from build123d import *

# Parameters (mm, degrees)
CROQUIS2_W              = 290
CROQUIS2_H              = 130
SALIENTE_EXTRUIR1_DEPTH = 5
CROQUIS3_W              = 90
CROQUIS3_H              = 5
CORTAR_EXTRUIR1_DEPTH   = 159.981130956
CROQUIS4_W              = 20.5
CROQUIS4_H              = 25.7
CORTAR_EXTRUIR2_DEPTH   = 4
CROQUIS5_R              = 1.25
CORTAR_EXTRUIR3_DEPTH   = 4
CROQUIS6_W              = 92
CROQUIS6_H              = 104.5
CORTAR_EXTRUIR4_DEPTH   = 3
CROQUIS7_W              = 100
CROQUIS7_H              = 8.5
CORTAR_EXTRUIR5_DEPTH   = 159.981130956
CROQUIS8_R              = 2
CORTAR_EXTRUIR6_DEPTH   = 159.981130956
CROQUIS9_R              = 3.75
CORTAR_EXTRUIR7_DEPTH   = 2
CROQUIS10_W             = 122
CROQUIS10_H             = 82
CORTAR_EXTRUIR8_DEPTH   = 4
CROQUIS13_R             = 1.4
CORTAR_EXTRUIR9_DEPTH   = 3
CROQUIS14_R             = 1.4
CORTAR_EXTRUIR10_DEPTH  = 3
SALIENTE_EXTRUIR2_DEPTH = 1
CROQUIS16_R             = 1.375
CORTAR_EXTRUIR11_DEPTH  = 159.95282319


with BuildPart() as part:
    # Croquis2 → Saliente-Extruir1 (new body)
    with BuildSketch(Plane(origin=(0, 0, 0), x_dir=(1, 0, 0), z_dir=(0, 1, 0))):
        Rectangle(CROQUIS2_W, CROQUIS2_H)
    extrude(amount=SALIENTE_EXTRUIR1_DEPTH)

    # Croquis3 → Cortar-Extruir1 (cut, through all)
    with BuildSketch(Plane(origin=(0, 5, 0), x_dir=(1, 0, 0), z_dir=(0, 1, 0))):
        with Locations((92.5, -57.5)):
            Rectangle(CROQUIS3_W, CROQUIS3_H)
        with Locations((-92.5, -57.5)):
            Rectangle(CROQUIS3_W, CROQUIS3_H)
        with Locations((92.5, 57.5)):
            Rectangle(CROQUIS3_W, CROQUIS3_H)
        with Locations((-92.5, 57.5)):
            Rectangle(CROQUIS3_W, CROQUIS3_H)
    extrude(amount=-CORTAR_EXTRUIR1_DEPTH, mode=Mode.SUBTRACT)

    # Croquis4 → Cortar-Extruir2 (cut)
    with BuildSketch(Plane(origin=(0, 5, 0), x_dir=(1, 0, 0), z_dir=(0, 1, 0))):
        with Locations((-120.05, -1.95)):
            Rectangle(CROQUIS4_W, CROQUIS4_H)
    extrude(amount=-CORTAR_EXTRUIR2_DEPTH, mode=Mode.SUBTRACT)

    # Croquis5 → Cortar-Extruir3 (cut)
    with BuildSketch(Plane(origin=(0, 1, 0), x_dir=(1, 0, 0), z_dir=(0, 1, 0))):
        with Locations(Location((-127.8, 8.4, 0), (0, 0, 270))):
            Circle(CROQUIS5_R)
        with Locations(Location((-112.3, 8.4, 0), (0, 0, 90))):
            Circle(CROQUIS5_R)
        with Locations(Location((-112.3, -12.3, 0), (0, 0, 270))):
            Circle(CROQUIS5_R)
        with Locations(Location((-127.8, -12.3, 0), (0, 0, 90))):
            Circle(CROQUIS5_R)
    extrude(amount=-CORTAR_EXTRUIR3_DEPTH, mode=Mode.SUBTRACT)

    # Croquis6 → Cortar-Extruir4 (cut)
    with BuildSketch(Plane(origin=(0, 5, 0), x_dir=(1, 0, 0), z_dir=(0, 1, 0))):
        with Locations((85.8, 0)):
            Rectangle(CROQUIS6_W, CROQUIS6_H)
    extrude(amount=-CORTAR_EXTRUIR4_DEPTH, mode=Mode.SUBTRACT)

    # Croquis7 → Cortar-Extruir5 (cut, through all)
    with BuildSketch(Plane(origin=(0, 5, 0), x_dir=(1, 0, 0), z_dir=(0, 1, 0))):
        with Locations((-50, -46.25)):
            Rectangle(CROQUIS7_W, CROQUIS7_H)
        with Locations((-50, 46.25)):
            Rectangle(CROQUIS7_W, CROQUIS7_H)
    extrude(amount=-CORTAR_EXTRUIR5_DEPTH, mode=Mode.SUBTRACT)

    # Croquis8 → Cortar-Extruir6 (cut, through all)
    with BuildSketch(Plane(origin=(0, 5, 0), x_dir=(1, 0, 0), z_dir=(0, 1, 0))):
        with Locations(Location((-140, 50, 0), (0, 0, 270))):
            Circle(CROQUIS8_R)
        with Locations(Location((140, 50, 0), (0, 0, 90))):
            Circle(CROQUIS8_R)
        with Locations(Location((140, -50, 0), (0, 0, 270))):
            Circle(CROQUIS8_R)
        with Locations(Location((-140, -50, 0), (0, 0, 90))):
            Circle(CROQUIS8_R)
    extrude(amount=-CORTAR_EXTRUIR6_DEPTH, mode=Mode.SUBTRACT)

    # Croquis9 → Cortar-Extruir7 (cut)
    with BuildSketch(Plane(origin=(0, 5, 0), x_dir=(1, 0, 0), z_dir=(0, 1, 0))):
        with Locations(Location((-140, 50, 0), (0, 0, 270))):
            Circle(CROQUIS9_R)
        with Locations(Location((-140, -50, 0), (0, 0, 90))):
            Circle(CROQUIS9_R)
        with Locations(Location((140, -50, 0), (0, 0, 270))):
            Circle(CROQUIS9_R)
        with Locations(Location((140, 50, 0), (0, 0, 90))):
            Circle(CROQUIS9_R)
    extrude(amount=-CORTAR_EXTRUIR7_DEPTH, mode=Mode.SUBTRACT)

    # Croquis10 → Cortar-Extruir8 (cut)
    with BuildSketch(Plane(origin=(0, 5, 0), x_dir=(1, 0, 0), z_dir=(0, 1, 0))):
        with Locations((-46.8, 0)):
            Rectangle(CROQUIS10_W, CROQUIS10_H)
    extrude(amount=-CORTAR_EXTRUIR8_DEPTH, mode=Mode.SUBTRACT)

    # Croquis13 → Cortar-Extruir9 (cut)
    with BuildSketch(Plane(origin=(0, 1, 0), x_dir=(1, 0, 0), z_dir=(0, 1, 0))):
        with Locations(Location((-104.3, 37.5, 0), (0, 0, 270))):
            Circle(CROQUIS13_R)
        with Locations(Location((10.7, 37.5, 0), (0, 0, 90))):
            Circle(CROQUIS13_R)
        with Locations(Location((10.7, -37.5, 0), (0, 0, 270))):
            Circle(CROQUIS13_R)
        with Locations(Location((-104.3, -37.5, 0), (0, 0, 90))):
            Circle(CROQUIS13_R)
    extrude(amount=-CORTAR_EXTRUIR9_DEPTH, mode=Mode.SUBTRACT)

    # Croquis14 → Cortar-Extruir10 (cut)
    with BuildSketch(Plane(origin=(0, 1, 0), x_dir=(1, 0, 0), z_dir=(0, 1, 0))):
        with Locations(Location((-104.3, -37.5, 0), (0, 0, 90))):
            Circle(CROQUIS14_R)
        with Locations(Location((-104.3, 37.5, 0), (0, 0, 270))):
            Circle(CROQUIS14_R)
        with Locations(Location((-11.3, 37.5, 0), (0, 0, 90))):
            Circle(CROQUIS14_R)
        with Locations(Location((-11.3, -37.5, 0), (0, 0, 90))):
            Circle(CROQUIS14_R)
    extrude(amount=-CORTAR_EXTRUIR10_DEPTH, mode=Mode.SUBTRACT)

    # Croquis15 → Saliente-Extruir2 (add)
    with BuildSketch(Plane(origin=(0, 5, 0), x_dir=(1, 0, 0), z_dir=(0, 1, 0))):
        with BuildLine():
            Line((-107.8, 42), (-100.783894533, 42))
            Line((-100.783894533, 42), (-100.783894533, 41))
            Line((-100.783894533, 41), (-107.8, 41))
            Line((-107.8, 41), (-107.8, 34.318360621))
            Line((-107.8, 34.318360621), (-108.8, 34.318360621))
            Line((-108.8, 34.318360621), (-108.8, 41))
            ThreePointArc((-108.8, 41), (-108.507106781, 41.707106781), (-107.8, 42))
        make_face()
        with BuildLine():
            Line((15.2, 41), (15.2, 34.318360621))
            Line((15.2, 34.318360621), (14.2, 34.318360621))
            Line((14.2, 34.318360621), (14.2, 41))
            Line((14.2, 41), (7.183894533, 41))
            Line((7.183894533, 41), (7.183894533, 42))
            Line((7.183894533, 42), (14.2, 42))
            ThreePointArc((14.2, 42), (14.907106781, 41.707106781), (15.2, 41))
        make_face()
        with BuildLine():
            Line((14.2, -42), (7.183894533, -42))
            Line((7.183894533, -42), (7.183894533, -41))
            Line((7.183894533, -41), (14.2, -41))
            Line((14.2, -41), (14.2, -34.318360621))
            Line((14.2, -34.318360621), (15.2, -34.318360621))
            Line((15.2, -34.318360621), (15.2, -41))
            ThreePointArc((15.2, -41), (14.907106781, -41.707106781), (14.2, -42))
        make_face()
        with BuildLine():
            Line((-108.8, -41), (-108.8, -34.318360621))
            Line((-108.8, -34.318360621), (-107.8, -34.318360621))
            Line((-107.8, -34.318360621), (-107.8, -41))
            Line((-107.8, -41), (-100.783894533, -41))
            Line((-100.783894533, -41), (-100.783894533, -42))
            Line((-100.783894533, -42), (-107.8, -42))
            ThreePointArc((-107.8, -42), (-108.507106781, -41.707106781), (-108.8, -41))
        make_face()
    extrude(amount=SALIENTE_EXTRUIR2_DEPTH)

    # Croquis16 → Cortar-Extruir11 (cut, through all)
    with BuildSketch(Plane(origin=(0, 2, 0), x_dir=(1, 0, 0), z_dir=(0, 1, 0))):
        with Locations(Location((50.3, 40, 0), (0, 0, 270))):
            Circle(CROQUIS16_R)
        with Locations(Location((50.3, -46, 0), (0, 0, 270))):
            Circle(CROQUIS16_R)
        with Locations(Location((108.3, 40, 0), (0, 0, 270))):
            Circle(CROQUIS16_R)
        with Locations(Location((108.3, -46, 0), (0, 0, 270))):
            Circle(CROQUIS16_R)
    extrude(amount=-CORTAR_EXTRUIR11_DEPTH, mode=Mode.SUBTRACT)


solid = part.part
Can you work these out from the model? Positions are in its coordinate system, mm. A direction names the side the tool comes from. Coordinates: 2 decimals unless noted, no trailing zeros. Loops run counter-clockwise (first coordinate to the right, second up) from the corner with the lowest first, then second, coordinate; pieces in that order, holes last. Notation, with made-up numbers: M 83.25,-24 L 117.25,-24 A33 cw 117.25,10 Z; hole C 17,60.5 d2. An arc over 180 degrees is marked long. Return JSON: item names as keys, results as strings. Group by question number.
Item 1: On a 3-axis mill with a long thin cutter (end or side, diameter ignored), from which of +Z, -Z, +X, -X, +Y, -Y can I reach the whole of each face in a straight line? I mean faces 1 (the flat face through (-107.8, 3, 1)), 2 (the flat face through (-2, 2, -65)), 3 (the flat face through (-100, 3, 46)). Say none if no direction works.
Item 2: Imagine slicing it at C-C (z = -24.5). Please give me the cut outline in (x, y).
Item 3: Imagine slicing it at A-A (x = -16). Please give me the cut outline in (y, z), and give its area (3 significant figures).
Item 4: Imagine slicing it at B-B (z = 3.5). Please give me the cut outline in (x, y), and give its area (3 significant figures).
Item 5: I'm going to push flat-ended pins straight in: pin 1 Ø4.5 at (x, z) = (-104.3, 37.5) entering from -Y; pin 2 Ø0.8 at (y, z) = (5.5, 41.5) entering from -X (3 decimals); pin 3 Ø3.5 at (x, z) = (-104.3, -37.5) entering from +Y; pin 4 Ø7 at (x, z) = (-140, -50) entering from +Y. Where does each tip first touch, or does it pass through?
Item 6: If I drill on L1, parallel to Z at x = -13, y = 0.6; L2, parallel to Z at x = 110, y = 2.15; L3, parallel to X at y = 0.8, z = 57, over which ranges is the centre line in solid material (lowest first)? Write a range as from..to.
Verdict:
{
 "1": {"face 1": "+Y", "face 2": "-Z, +X, -X, +Y, -Y", "face 3": "+Y, -Y"},
 "2": {"outline": "M -145,0 L 145,0 L 145,5 L 131.8,5 L 131.8,2 L 39.8,2 L 39.8,5 L 14.2,5 L 14.2,1 L -107.8,1 L -107.8,5 L -145,5 Z"},
 "3": {"outline": "M 0,-65 L 5,-65 L 5,-50.5 L 0,-50.5 Z; M 0,-42 L 5,-42 L 5,-41 L 1,-41 L 1,41 L 5,41 L 5,42 L 0,42 Z; M 0,50.5 L 5,50.5 L 5,65 L 0,65 Z", "area": "237 mm^2"},
 "4": {"outline": "M -145,0 L 145,0 L 145,5 L 131.8,5 L 131.8,2 L 39.8,2 L 39.8,5 L 14.2,5 L 14.2,1 L -107.8,1 L -107.8,5 L -109.8,5 L -109.8,1 L -130.3,1 L -130.3,5 L -145,5 Z", "area": "604 mm^2"},
 "5": {"pin 1": "stops at y = 0", "pin 2": "stops at x = -108.795", "pin 3": "stops at y = 1", "pin 4": "stops at y = 3"},
 "6": {"L1": "z = -65..-50.5, -42..42, 50.5..65", "L2": "z = -65..-60, -55..-52.25, 52.25..55, 60..65", "L3": "x = -145..-137.5, -47.5..47.5, 137.5..145"}
}
